Build history of the part. All positions in model axes, mm. A direction names the side the tool comes from. Give positions to 0.01 mm unless a question says otherwise; leave off trailing zeros. Write each loop counter-clockwise with the first axis right and the second up, starting at its lowest first coordinate (ties: lowest second). Pieces come first, ordered by that corner, then holes.
Autodesk Fusion 360 part; units mm, degrees
sketch "Sketch1" plane through (0, 0, 0) normal (0, 0, 1) x (1, 0, 0)
  line L0 (0, 0) -> (27, 0)
  line L1 (27, 0) -> (27, -13)
  line L2 (27, -13) -> (0, -13)
  line L3 (0, -13) -> (0, 0)
  dimension "d1" = 27
  dimension "d2" = 13
extrude "Extrude1" add sketch "Sketch1" along normal blind 0.5
extrude "Extrude2" add 1 faces at (9, -8.6667, 0.5) along direction (0, 0, 1) blind 1.5
sketch "Sketch2" plane through (0, 0, 2) normal (0, 0, 1) x (-1, 0, 0)
  line L0 (0, 13) -> (-27, 13)
  line L1 (-27, 13) -> (-27, 0)
  line L2 (-27, 0) -> (0, 0)
  line L3 (0, 0) -> (0, 13)
  line L4 (0, 13) -> (-22, 13)
  line L5 (-22, 13) -> (-22, -5)
  line L6 (-22, -5) -> (0, -5)
  line L7 (0, -5) -> (0, 13)
  dimension "d7" = 22
  dimension "d8" = 18
extrude "Extrude3" add sketch "Sketch2" along normal blind 21 contours L0 L2 L3 L4 L5 L7 | L2 L5 L6 L7
extrude "Extrude4" add 1 faces at (16.3333, 0, 0.6667) along direction (0, 1, 0) blind 5
sketch "Sketch3" plane through (0, -13, 0) normal (0, -1, 0) x (1, 0, 0)
  line L0 (0, 0) -> (27, 0)
  line L1 (27, 0) -> (27, 2)
  line L2 (27, 2) -> (22, 2)
  line L3 (22, 2) -> (22, 23)
  line L4 (22, 23) -> (0, 23)
  line L5 (0, 23) -> (0, 0)
  circle A0 centre (11, 11.5) radius 7.5
  line L6 (0, 2) -> (22, 2) construction
  line L7 (27.4979, -2) -> (0.4979, -2) construction
  line L8 (-1.5021, 4) -> (29.4979, 4) construction
  dimension "d13" = 15
  dimension "d14" = 6
  dimension "d15" = 7.5
  dimension "d16" = 11
extrude "Extrude5" cut sketch "Sketch3" against normal blind 15 contours A0
fillet "Fillet1" radius 11 2 edges at (22, -4, 23) (0, -4, 23)
fillet "Fillet2" radius 2 1 edges at (4.0075, -13, 14.2121)
(1) Mould opens along Z. For faces 4 (the face through (27, -4, 1)), 5 (the face through (9.37, -4.59, 4.18)), 6 (the face through (13, -4, 0)) say: +Z half, -Z half, draft (parallel to the pull), parting line (faces both ways), or undercut.
(2) Drop flat-ended pins along their axis: pin 1 (3 mm diameter, centred on y = -4.5, z = 8.5, fed in from +X); pin 2 (4 mm diameter, centred on x = 25.5, y = -7, fed in from +Z); pin 3 (3 mm diameter, centred on x = 14.5, z = 8.5, fed in from -Y). Give the stop position or say it passes through.
(3) Saw through at C-C, the plane x = 22.5. List the corners of the cut face in (y, z), plus the area to 3 significant figures.
(4) Probe line 1 (Z direction, x = 11, y = -0.75); line 2 (X direction, y = -1.5, z = 12.75); line 3 (Z direction, x = 22.25, y = -7.25). List the from-to ranges inside material, lowest first.
(5) Saw through at B-B, the plane z = 11.5. List the corners of the cut face in (x, y), plus the area to 3 significant figures.
(6) 3-axis set-ups, long thin cutter, end or side, ignore diameter. For faces 1 (the face through (0, -4, 6)), 2 (the face through (22, -4, 7)), 3 (the face through (11, 2, 12)): which of +Z, -Z, +X, -X, +Y, -Y reach the whole face in a straight line?
Computed values:
1. face 4: draft
1. face 5: undercut
1. face 6: -Z half
2. pin 1: stops at x = 22
2. pin 2: stops at z = 2
2. pin 3: stops at y = 2
3. outline: (-13, 0) - (5, 0) - (5, 2) - (-13, 2) - close
3. area: 36.0 mm2
4. line 1: z = 0 to 4, 19 to 23
4. line 2: x = 0.03 to 3.6, 18.4 to 21.97
4. line 3: z = 0 to 2
5. outline: (0, -13) - (1.5, -13) arc R2 ccw to (3.5, -11) - (3.5, 2) - (18.5, 2) - (18.5, -11) arc R2 ccw to (20.5, -13) - (22, -13) - (22, 5) - (0, 5) - close
5. area: 169 mm2
6. face 1: +Z, -Z, -X, +Y, -Y
6. face 2: +Z, +X, +Y, -Y
6. face 3: -Y
